Geometry check sheet. Reference: the model listing, model coordinates, mm. Face numbers are marked on the shaded views. A direction names the side the tool comes from. Coordinates: 2 decimals unless noted, no trailing zeros. Order: outer loops, then holes, each group sorted by start corner. A loop starts at its lowest first (then second) coordinate and runs counter-clockwise, first axis right, second up. Notation, with made-up numbers: (-33, 28) - (9, 28) arc R12 cw to (9, 32) - close; hole circle Ø2 at (-14.75, -26.5). An arc over 180 degrees is marked (long way). One line per item, written item: value. Start each with the question number.
```python
from build123d import *

# Parameters (mm, degrees)
BOSS_EXTRUDE1_DEPTH              = 2
CUT_EXTRUDE2_REACH               = 30.124
CUT_EXTRUDE2_START               = 15
SKETCH3_W                        = 6.7
SKETCH3_H                        = 0.8
CUT_EXTRUDE3_REACH               = 23.248
CUT_EXTRUDE3_OFFSET_FROM_SURFACE = 10
SKETCH4_W                        = 2.662765864
SKETCH4_H                        = 0.8
FILLET1_R                        = 0.4


with BuildPart() as part:
    # Sketch1 → Boss-Extrude1 (new, symmetric)
    with BuildSketch(Plane.XY):
        with BuildLine():
            Line((1.77938838, -1.075884724), (2.07938838, -1.075884724))
            Line((2.07938838, -1.075884724), (2.07938838, 10.209972433))
            ThreePointArc((2.07938838, 10.209972433), (1.58135883, 11.074857205), (0.583337044, 11.078265628))
            Line((0.583337044, 11.078265628), (-4.380611082, 8.242388166))
            ThreePointArc((-4.380611082, 8.242388166), (-4.45031283, 8.2134957), (-4.525019051, 8.202908502))
            Line((-4.525019051, 8.202908502), (-6.525019051, 8.173522453))
            Line((-6.525019051, 8.173522453), (-6.52061162, 7.873554831))
            Line((-6.52061162, 7.873554831), (-4.52061162, 7.902940879))
            ThreePointArc((-4.52061162, 7.902940879), (-4.371199177, 7.924115276), (-4.231795681, 7.981900208))
            Line((-4.231795681, 7.981900208), (0.619506411, 10.753423582))
            ThreePointArc((0.619506411, 10.753423582), (1.393268277, 10.750781047), (1.77938838, 10.080239717))
            Line((1.77938838, 10.080239717), (1.77938838, -1.075884724))
        make_face()
    extrude(amount=BOSS_EXTRUDE1_DEPTH, both=True)

    # Cut-Extrude2: up to this plane
    cut_extrude2_end = Plane(origin=(0.619506411, 10.753423582, 2), z_dir=(-0.49605133620388303, 0.8682931946355115, 0))
    # Sketch3 → Cut-Extrude2 (cut, up to the surface)
    with BuildSketch(Plane(origin=(0, 0, 0), x_dir=(1, 0, 0), z_dir=(0, 1, 0)).offset(CUT_EXTRUDE2_START), mode=Mode.PRIVATE) as cut_extrude2_sk1:
        with Locations((-1.27061162, 0)):
            Rectangle(SKETCH3_W, SKETCH3_H)
    cut_extrude2_tool1 = split(extrude(cut_extrude2_sk1.sketch, amount=-CUT_EXTRUDE2_REACH, mode=Mode.PRIVATE), bisect_by=cut_extrude2_end, keep=Keep.BOTH, mode=Mode.PRIVATE)
    add(cut_extrude2_tool1.solids().sort_by_distance((-1.270612, 15, 0))[0], mode=Mode.SUBTRACT)

    # Cut-Extrude3: up to this face of the body (flat: up to its plane, moved by the offset)
    cut_extrude3_end = Plane(part.part.faces().sort_by_distance((1.92938838, -1.075884724, 0))[0]).offset(-CUT_EXTRUDE3_OFFSET_FROM_SURFACE)
    # Sketch4 → Cut-Extrude3 (cut, up to the picked face)
    with BuildSketch(Plane(origin=(-4.479253053, 7.840529112, 0), x_dir=(0.8682931946355115, 0.49605133620388303, 0), z_dir=(-0.49605133620388303, 0.8682931946355115, 0)), mode=Mode.PRIVATE) as cut_extrude3_sk1:
        with Locations((7.203546269, 0)):
            Rectangle(SKETCH4_W, SKETCH4_H)
    cut_extrude3_tool1 = split(extrude(cut_extrude3_sk1.sketch, amount=-CUT_EXTRUDE3_REACH, mode=Mode.PRIVATE), bisect_by=cut_extrude3_end, keep=Keep.BOTH, mode=Mode.PRIVATE)
    add(cut_extrude3_tool1.solids().sort_by(Axis((1.775537, 11.413858, 0), (0.49605133620388303, -0.8682931946355115, 0)))[0], mode=Mode.SUBTRACT)

    # Fillet1
    fillet1_edges = [part.edges().sort_by_distance(p)[0] for p in [
        (-4.62061162, 8.051487767, -0.4),
        (-4.62061162, 8.051487767, 0.4),
        (1.92938838, 8.924115276, -0.4),
        (1.92938838, 8.924115276, 0.4),
    ]]
    fillet(fillet1_edges, radius=FILLET1_R - 0.0001)  # a hair under: the kernel refuses the full size


solid = part.part
```
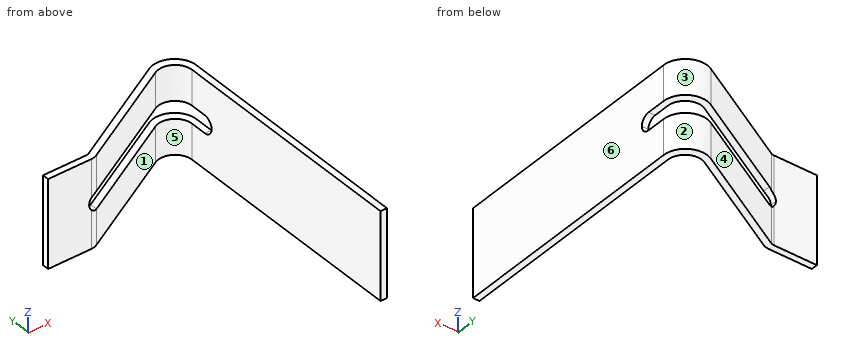
Q1. Set-up check for the marked faces 1 and 2: record each of +Z, -Z, +X, -X, +Y, -Y from which the full face is reachable in a straight line by a thin tool's end or side.
Q2. Cross-section at C-C, the plane y = 6.25. Enter the section's corners in (x, z).
Q3. Gauge pin test, flat end, axial feed: P1, Ø1.5, axis at y = 2.5, z = 0.5, coming from the -X side. Record the tip position at first contact, or that the pin passes through.
Q4. Cross-section at B-B, the plane x = 0.25. Enter the section's corners in (y, z).
Q5. Cross-section at D-D, the plane x = 1.25. Enter the section's corners in (y, z).
Q6. Release check for a two-part mould opening along X. For the marked faces 3, 4, 5 and 6 record: released by +X, released by -X, zero draft, split by the parting line, or undercut.
Q7. Material ranges on probe 1 along X at (y, z) = (5, -1.2); probe 2 along X at (y, z) = (10.25, -0.6); probe 3 along X at (y, z) = (9.75, 1.5), recorded low to high.
Q8. Cross-section at A-A, the plane z = -1. Enter the section's corners in (x, y).
Check result:
1. face 1: +Z, -Z, -Y
1. face 2: +Z, -Z, +Y
2. outline: (1.78, -2) - (2.08, -2) - (2.08, 2) - (1.78, 2) - close
3. P1: stops at x = 1.78
4. outline: (10.54, -2) - (10.89, -2) - (10.89, -0.4) - (10.54, -0.4) - close; (10.54, 0.4) - (10.89, 0.4) - (10.89, 2) - (10.54, 2) - close
5. outline: (10.82, -2) - (11.2, -2) - (11.2, -0.4) - (10.82, -0.4) - close; (10.82, 0.4) - (11.2, 0.4) - (11.2, 2) - (10.82, 2) - close
6. face 3: split by the parting line
6. face 4: released by -X
6. face 5: undercut
6. face 6: released by +X
7. probe 1: x = 1.78 to 2.08
7. probe 2: x = -0.87 to -0.26, 1.76 to 2.08
7. probe 3: x = -1.74 to -1.14, 1.78 to 2.08
8. outline: (-6.53, 8.17) - (-6.52, 7.87) - (-4.52, 7.9) arc R0.6 ccw to (-4.23, 7.98) - (0.62, 10.75) arc R0.78 cw to (1.78, 10.08) - (1.78, -1.08) - (2.08, -1.08) - (2.08, 10.21) arc R1 ccw to (0.58, 11.08) - (-4.38, 8.24) arc R0.3 cw to (-4.53, 8.2) - close
